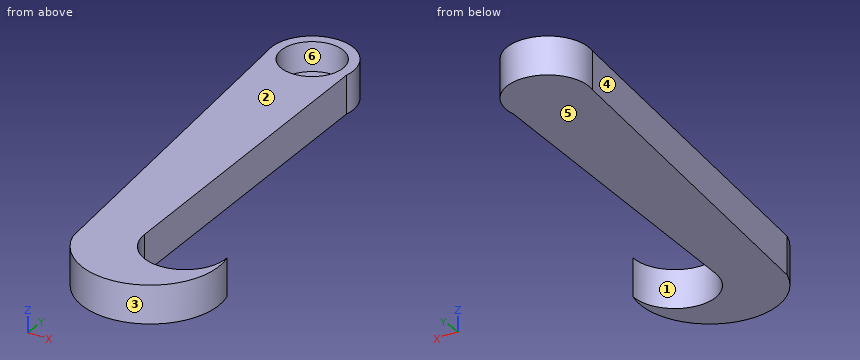
from build123d import *

# Parameters (mm, degrees)
SKETCH_1_R          = 14
EXTRUDE_1_DEPTH     = 13
SKETCH_3_R          = 4
CUT_EXTRUDE_2_DEPTH = 10
EXTRUDE_START       = -13
EXTRUDE_3_DEPTH     = 13
SKETCH_7_R          = 10.6
CUT_EXTRUDE_3_DEPTH = 10


with BuildPart() as part:
    # 스케치1 → 보스-돌출1 (new body)
    with BuildSketch(Plane.XY):
        with Locations(Location((0, 0, 0), (0, 0, 180))):
            Circle(SKETCH_1_R)
    extrude(amount=EXTRUDE_1_DEPTH)

    # 스케치3 → 컷-돌출2 (cut)
    with BuildSketch(Plane.XY.offset(13)):
        Circle(SKETCH_3_R)
    extrude(amount=-CUT_EXTRUDE_2_DEPTH, mode=Mode.SUBTRACT)

    # 스케치6 → 보스-돌출3 (add)
    with BuildSketch(Plane.XY.offset(13).offset(EXTRUDE_START)):
        with BuildLine():
            Line((13.735578357, -2.708115061), (17.539668143, -115.708115061))
            ThreePointArc((17.539668143, -115.708115061), (32.332669837, -129.214149758), (45.486033392, -114.10670459))
            ThreePointArc((45.486033392, -114.10670459), (29.938586036, -143.187708961), (0.608578272, -128.115264599))
            Line((0.608578272, -128.115264599), (-13.64899727, -3.115264599))
            ThreePointArc((-13.64899727, -3.115264599), (0.208126783, -13.998452887), (13.735578357, -2.708115061))
        make_face()
    extrude(amount=EXTRUDE_3_DEPTH)

    # 스케치7 → 컷-돌출3 (cut)
    with BuildSketch(Plane.XY.offset(13)):
        Circle(SKETCH_7_R)
    extrude(amount=-CUT_EXTRUDE_3_DEPTH, mode=Mode.SUBTRACT)


solid = part.part
The model under review builds one solid part; all positions refer to its coordinate system, in mm. Face numbers are marked on the shaded views. A direction names the side the tool comes from. Coordinates: 2 decimals unless noted, no trailing zeros. Write each loop counter-clockwise with the first axis right and the second up, starting at its lowest first coordinate (ties: lowest second). Pieces come first, ordered by that corner, then holes. Notation, with made-up numbers: (10.25, -14.5) - (42.25, -14.5) arc R21 cw to (42.25, -7.5) - close; hole circle Ø9 at (24.5, -20). An arc over 180 degrees is marked (long way). Answer as a JSON object with one key per item and string values. Group by question number.
1. Add section C-C (x = 2). Give the boundary of the cut face in (y, z), plus the area to 3 significant figures.
2. Clearance check with flat-ended pins moving along their axes: pin 1 Ø1 at (x, z) = (3.5, 5) entering from +Y; pin 2 Ø6 at (y, z) = (-12.5, 10.5) entering from -X; pin 3 Ø1.5 at (x, z) = (22, 2) entering from +Y. State where each tip first meets the part, or that it passes through.
3. Machinability: for the marked faces 5 and 6, which of the approach directions +Z, -Z, +X, -X, +Y, -Y give a long, thin tool a straight path to every point of the face, cutting with its end or side? Answer none if there is none.
4. Mouldability with a two-part tool opening along X and no side actions: class the marked faces 1, 2, 3 and 4 as pulls with the +X half, pulls with the -X half, needs draft (parallel to the pull), parting line crosses it, or undercut.
5. Add section A-A (y = 0). Give the boundary of the cut face in (x, z).
6. To check wall thickness, follow probe 1 along X at (y, z) = (5.5, 3.5); probe 2 along X at (y, z) = (-120, 3.75); probe 3 along X at (y, z) = (-37.5, 6.25). State the ranges of each line that lie inside material, in increasing order.
7. Add section D-D (x = 28). Give the boundary of the cut face in (y, z), plus the area to 3 significant figures.
8. Add section B-B (z = 5.5). Give the boundary of the cut face in (x, y), plus the area to 3 significant figures.
Findings:
{
 "1": {"outline": "(-131.45, 0) - (13.86, 0) - (13.86, 13) - (10.41, 13) - (10.41, 3) - (-10.41, 3) - (-10.41, 13) - (-131.45, 13) - close", "area": "1,680 mm²"},
 "2": {"pin 1": "y = 13.67", "pin 2": "x = -12.92", "pin 3": "y = -124.74"},
 "3": {"face 5": "-Z, +X, -X, +Y, -Y", "face 6": "+Z"},
 "4": {"face 1": "undercut", "face 2": "needs draft", "face 3": "parting line crosses it", "face 4": "pulls with the -X half"},
 "5": {"outline": "(-14, 0) - (14, 0) - (14, 13) - (10.6, 13) - (10.6, 3) - (-10.6, 3) - (-10.6, 13) - (-14, 13) - close"},
 "6": {"probe 1": "-12.87 to -9.06, 9.06 to 12.87", "probe 2": "-0.32 to 18.37, 44.7 to 46.43", "probe 3": "-9.73 to 14.91"},
 "7": {"outline": "(-143.7, 0) - (-128.78, 0) - (-128.78, 13) - (-143.7, 13) - close", "area": "194 mm²"},
 "8": {"outline": "(-13.65, -3.12) - (0.61, -128.12) arc R23.51 ccw to (45.49, -114.11) arc R14 cw (long way) to (17.54, -115.71) - (13.74, -2.71) arc R14 ccw (long way) to start; hole circle Ø21.2 at (0, 0)", "area": "3,420 mm²"}
}
